The listing builds one solid part. Answer for the finished solid, in the listing's coordinates (mm). Round coordinates to 2 decimals unless told otherwise and drop trailing zeros. One line per item, written item: value. Start each with the question number.
1. A straight line is drawn through the part: line 1 (X direction, y = 0.5, z = -72.5). Find the intervals that lie inside material, in ascending order.
2. Flat-ended cylindrical pins translate along their axes: P1, Ø12, axis at x = 35.5, z = -26.5, coming from the -Y side; P2, Ø2, axis at x = 3.302, z = -73.025, coming from the +Y side. Find the tip coordinate at first contact, or state that the pin passes through.
3. For a pull along Z with two mould halves and no side action, classify faces 1 (the cylindrical face through (69.326, 0.789, -72.241)), 2 (the flat face through (0, 1, -39)), 3 (the flat face through (35, 1, 0)) as released by +Z, released by -Z, zero draft, split by the parting line, or undercut.
Autodesk Inventor part; units mm, degrees
ref_plane "Work Plane1" through (0, 0, -38.735) normal (0, 0, 1) x (1, 0, 0)
ref_plane "Work Plane2" through (35.56, 0, -77.47) normal (-1, 0, 0) x (0, 0, 1)
ref_plane "YZ Plane" through (0, 0, 0) normal (1, 0, 0) x (0, 1, 0)
sketch "Sketch1" plane through (0, 0, 0) normal (0, 1, 0) x (-1, 0, 0)
  line L0 (0, 0) -> (-71.12, 0)
  line L1 (-71.12, 0) -> (-71.12, -77.47)
  line L2 (-71.12, -77.47) -> (0, -77.47)
  line L3 (0, -77.47) -> (0, 0)
  dimension "d0" = 71.12
  dimension "d1" = 77.47
extrude "Extrusion1" add sketch "Sketch1" along normal blind 1.6
sketch "Sketch2" plane through (0, 1.6, 0) normal (0, 1, 0) x (1, 0, 0)
  line L0 (67.818, 4.445) -> (3.302, 4.445) construction
  line L1 (3.302, 4.445) -> (3.302, 73.025) construction
  line L2 (3.302, 73.025) -> (67.818, 73.025) construction
  line L3 (67.818, 73.025) -> (67.818, 4.445) construction
  line L4 (0, 0) -> (71.12, 0) construction
  line L5 (35.56, 0) -> (35.56, 77.47) construction
  line L6 (71.12, 77.47) -> (0, 77.47) construction
  line L7 (67.818, 73.025) -> (3.302, 4.445) construction
  point P0 (35.56, 38.735)
  dimension "d4" = 68.58
  dimension "d5" = 64.516
hole "Hole1" at (3.302, 1.6, -73.025) at (67.818, 1.6, -4.445) at (67.818, 1.6, -73.025) direction (0, -1, 0) diameter 3.4 end through all
ref_plane "Work Plane1" through (0, 0, -38.735) normal (0, 0, 1) x (1, 0, 0)
ref_plane "Work Plane2" through (35.56, 0, -77.47) normal (-1, 0, 0) x (0, 0, 1)
properties part number "PCB" material "Copper"
Answer list:
1. line 1: x = 0 to 1.69, 4.92 to 66.2, 69.43 to 71.12
2. P1: stops at y = 0
2. P2: passes through
3. face 1: undercut
3. face 2: zero draft
3. face 3: released by +Z
